Verification items for the finished model (mm, model axes). Face numbers are marked on the shaded views. Give positions to 0.01 mm unless a question says otherwise; leave off trailing zeros. Write each loop counter-clockwise with the first axis right and the second up, starting at its lowest first coordinate (ties: lowest second). Pieces come first, ordered by that corner, then holes. Notation, with made-up numbers: M 3,89 L 36,89 A19 cw 36,122 Z; hole C 85,6.5 d4. An arc over 180 degrees is marked long. Write item = value, one per line.
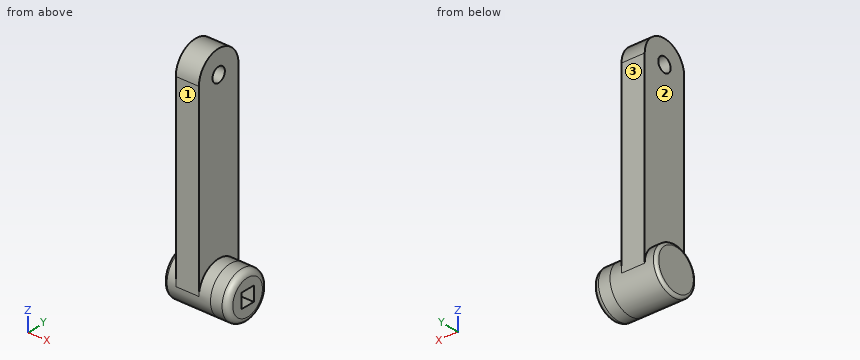
from build123d import *

# Parameters (mm, degrees)
SKETCH1_R           = 10.16
BOSS_EXTRUDE1_DEPTH = 10.16
FILLET1_R           = 1.27
BOSS_EXTRUDE2_DEPTH = 5.08
SKETCH3_R           = 10.16
BOSS_EXTRUDE3_DEPTH = 7.62
FILLET2_R           = 2.54
SKETCH4_W           = 6.35
SKETCH4_H           = 6.35
CUT_EXTRUDE1_DEPTH  = 25.4
SKETCH5_R           = 3.175
CUT_EXTRUDE2_DEPTH  = 16.24


with BuildPart() as part:
    # Sketch1 → Boss-Extrude1 (new body, symmetric)
    with BuildSketch(Plane(origin=(0, 0, 0), x_dir=(0, 0, -1), z_dir=(1, 0, 0))):
        Circle(SKETCH1_R)
    extrude(amount=BOSS_EXTRUDE1_DEPTH, both=True)

    # Fillet1
    fillet1_edges = [part.edges().sort_by_distance(p)[0] for p in [
        (-10.16, 0, 10.16),
    ]]
    fillet(fillet1_edges, radius=FILLET1_R)

    # Sketch2 → Boss-Extrude2 (add, symmetric)
    with BuildSketch(Plane(origin=(0, 0, 0), x_dir=(0, 0, -1), z_dir=(1, 0, 0))):
        with BuildLine():
            Line((-81.28, 10.16), (0, 10.16))
            ThreePointArc((0, 10.16), (10.16, 0), (0, -10.16))
            Line((0, -10.16), (-81.28, -10.16))
            ThreePointArc((-81.28, -10.16), (-91.44, 0), (-81.28, 10.16))
        make_face()
    extrude(amount=BOSS_EXTRUDE2_DEPTH, both=True)

    # Sketch3 → Boss-Extrude3 (add)
    with BuildSketch(Plane(origin=(10.16, 0, 0), x_dir=(0, 0, -1), z_dir=(1, 0, 0))):
        Circle(SKETCH3_R)
    extrude(amount=BOSS_EXTRUDE3_DEPTH)

    # Fillet2
    fillet2_edges = [part.edges().sort_by_distance(p)[0] for p in [
        (17.78, 0, 10.16),
    ]]
    fillet(fillet2_edges, radius=FILLET2_R)

    # Sketch4 → Cut-Extrude1 (cut)
    with BuildSketch(Plane(origin=(17.78, 0, 0), x_dir=(0, 0, -1), z_dir=(1, 0, 0))):
        Rectangle(SKETCH4_W, SKETCH4_H)
    extrude(amount=-CUT_EXTRUDE1_DEPTH, mode=Mode.SUBTRACT)

    # Sketch5 → Cut-Extrude2 (cut, through all)
    with BuildSketch(Plane(origin=(5.08, 0, 0), x_dir=(0, 0, -1), z_dir=(1, 0, 0))):
        with Locations((-81.28, 0)):
            Circle(SKETCH5_R)
    extrude(amount=-CUT_EXTRUDE2_DEPTH, mode=Mode.SUBTRACT)


solid = part.part
1) Draft check along Y on the marked faces 1, 2 and 3. Enter one of: +Y half, -Y half, draft (parallel to the pull), parting line (faces both ways), or undercut.
From the geometry:
face_1 = -Y half
face_2 = draft
face_3 = +Y half
2) Cross-section at A-A on y = 0. Record the boundary of the cut face in (x, z) (3 decimals), plus the area to 3 significant figures.
From the geometry:
outline = M -10.16,-8.89 A1.27 ccw -8.89,-10.16 L 15.24,-10.16 A2.54 ccw 17.78,-7.62 L 17.78,-3.175 L -7.62,-3.175 L -7.62,3.175 L 17.78,3.175 L 17.78,7.62 A2.54 ccw 15.24,10.16 L 5.08,10.16 L 5.08,78.105 L -5.08,78.105 L -5.08,10.16 L -8.89,10.16 A1.27 ccw -10.16,8.89 Z; M -5.08,84.455 L 5.08,84.455 L 5.08,91.44 L -5.08,91.44 Z
area = 1,160 mm^2
3) Cross-section at C-C on x = 9. Record the boundary of the cut face in (y, z) (3 decimals), plus the area to 3 significant figures.
From the geometry:
outline = C 0,0 d20.32; hole M -3.175,-3.175 L 3.175,-3.175 L 3.175,3.175 L -3.175,3.175 Z
area = 284 mm^2
4) Material ranges on probe 1 along Y at (x, z) = (0, 81.28) (3 decimals); probe 2 along Z at (x, y) = (-1.75, 1.5) (3 decimals); probe 3 along X at (y, z) = (2.5, 64), recorded low to high. Write a range as from..to.
From the geometry:
probe_1 = -10.16..-3.175, 3.175..10.16
probe_2 = -10.049..-3.175, 3.175..78.482, 84.078..91.329
probe_3 = -5.08..5.08
5) Cross-section at B-B on x = -2.5. Record the boundary of the cut face in (y, z) (3 decimals), plus the area to 3 significant figures.
From the geometry:
outline = M -10.16,0 A10.16 ccw 10.16,0 L 10.16,81.28 A10.16 ccw -10.16,81.28 Z; hole M -3.175,-3.175 L 3.175,-3.175 L 3.175,3.175 L -3.175,3.175 Z; hole C 0,81.28 d6.35
area = 1,900 mm^2
6) Depth check by flat-ended pin: P1, Ø1.5, axis at y = 4.5, z = 22.5, coming from the -X side; P2, Ø6, axis at y = -1, z = 22, coming from the +X side; P3, Ø12, axis at x = 13, z = 14, coming from the +Y side. Enter the tip coordinate at first touch or a pass-through.
From the geometry:
P1 = -5.08
P2 = 5.08
P3 = 6.26
7) Cross-section at D-D on z = 25. Record the boundary of the cut face in (x, y).
From the geometry:
outline = M -5.08,-10.16 L 5.08,-10.16 L 5.08,10.16 L -5.08,10.16 Z
